Could you check a few things on this model? Use its own coordinates, in mm. Give positions to 0.01 mm unless a question says otherwise; leave off trailing zeros. Use a Markdown table: item, result. Add a question column.
```python
from build123d import *

# Parameters (mm, degrees)
SKETCH_1_W          = 350
SKETCH_1_H          = 310
SKETCH_1_R          = 1.95
SKETCH_1_R_2        = 9
EXTRUDE_1_DEPTH     = 1
SKETCH_2_R          = 2.1
SKETCH_2_R_2        = 1.6
SKETCH_2_R_3        = 11
SKETCH_2_R_4        = 1.5
SKETCH_2_W          = 10
SKETCH_2_H          = 10
CUT_EXTRUDE_1_DEPTH = 10
SKETCH_3_RX         = 29.354112179
SKETCH_3_RY         = 16.489205711
CUT_EXTRUDE_2_DEPTH = 8


with BuildPart() as part:
    # 草图1 → 凸台-拉伸1 (new body)
    with BuildSketch(Plane.XY):
        with Locations((175, 155)):
            Rectangle(SKETCH_1_W, SKETCH_1_H)
        with Locations((10, 300)):
            Circle(SKETCH_1_R, mode=Mode.SUBTRACT)
        with Locations((10, 230)):
            Circle(SKETCH_1_R, mode=Mode.SUBTRACT)
        with Locations((10, 40)):
            Circle(SKETCH_1_R, mode=Mode.SUBTRACT)
        with Locations((10, 10)):
            Circle(SKETCH_1_R, mode=Mode.SUBTRACT)
        with Locations((340, 300)):
            Circle(SKETCH_1_R, mode=Mode.SUBTRACT)
        with Locations((340, 230)):
            Circle(SKETCH_1_R, mode=Mode.SUBTRACT)
        with Locations((340, 40)):
            Circle(SKETCH_1_R, mode=Mode.SUBTRACT)
        with Locations((340, 10)):
            Circle(SKETCH_1_R, mode=Mode.SUBTRACT)
        with Locations((130, 10)):
            Circle(SKETCH_1_R, mode=Mode.SUBTRACT)
        with Locations((220, 10)):
            Circle(SKETCH_1_R, mode=Mode.SUBTRACT)
        with Locations((10, 160)):
            Circle(SKETCH_1_R, mode=Mode.SUBTRACT)
        with Locations((340, 160)):
            Circle(SKETCH_1_R, mode=Mode.SUBTRACT)
        with Locations((130, 162)):
            Circle(SKETCH_1_R, mode=Mode.SUBTRACT)
        with Locations((220, 162)):
            Circle(SKETCH_1_R, mode=Mode.SUBTRACT)
        with Locations((175, 280)):
            Circle(SKETCH_1_R_2, mode=Mode.SUBTRACT)
        with Locations((130, 182)):
            Circle(SKETCH_1_R, mode=Mode.SUBTRACT)
        with Locations((220, 182)):
            Circle(SKETCH_1_R, mode=Mode.SUBTRACT)
        with Locations((80, 240)):
            Circle(SKETCH_1_R, mode=Mode.SUBTRACT)
        with Locations((270, 240)):
            Circle(SKETCH_1_R, mode=Mode.SUBTRACT)
        with Locations((155, 280)):
            Circle(SKETCH_1_R, mode=Mode.SUBTRACT)
        with Locations((195, 280)):
            Circle(SKETCH_1_R, mode=Mode.SUBTRACT)
    extrude(amount=EXTRUDE_1_DEPTH)

    # 草图2 → 切除-拉伸1 (cut)
    with BuildSketch(Plane(origin=(0, 0, 0), x_dir=(-1, 0, 0), z_dir=(0, 0, -1))):
        with Locations((-130, 135)):
            Circle(SKETCH_2_R)
        with Locations((-220, 45)):
            Circle(SKETCH_2_R)
        with Locations((-220, 135)):
            Circle(SKETCH_2_R)
        with Locations((-130, 45)):
            Circle(SKETCH_2_R)
        with Locations((-153.079689783, 50)):
            Circle(SKETCH_2_R_2)
        with Locations((-175, 28.079689783)):
            Circle(SKETCH_2_R_2)
        with Locations((-196.920310217, 50)):
            Circle(SKETCH_2_R_2)
        with Locations((-175, 50)):
            Circle(SKETCH_2_R_3)
        with Locations((-150, 137)):
            Circle(SKETCH_2_R_4)
        with Locations((-135, 90)):
            Circle(SKETCH_2_R_3)
        with Locations((-200, 137)):
            Circle(SKETCH_2_R_4)
        with Locations((-113.079689783, 90)):
            Circle(SKETCH_2_R_2)
        with Locations((-135, 68.079689783)):
            Circle(SKETCH_2_R_2)
        with Locations((-135, 111.920310217)):
            Circle(SKETCH_2_R_2)
        with Locations((-175, 110)):
            Rectangle(SKETCH_2_W, SKETCH_2_H)
    extrude(amount=-CUT_EXTRUDE_1_DEPTH, mode=Mode.SUBTRACT)

    # 草图3 → 切除-拉伸2 (cut)
    with BuildSketch(Plane.XY.offset(1)):
        with Locations((175, 244.534964975)):
            Ellipse(SKETCH_3_RX, SKETCH_3_RY)
    extrude(amount=-CUT_EXTRUDE_2_DEPTH, mode=Mode.SUBTRACT)


solid = part.part
```
1) For pin 1 (4.5 mm diameter, centred on x = 220, y = 10, fed in from +Z), with a flat end and sliding along its axis, tell me the tip position at first contact or that it passes through.
2) Please list where these lines run through material, in increasing order: line 1 (Y direction, x = 340, z = 0.5); line 2 (X direction, y = 50.5, z = 0.95); line 3 (X direction, y = 160, z = 0.1). Write a range as from..to.
3) Suppose I cut it at A-A on z = 0.5. Count the separate pieces of the cut face and the enclosed holes in it, and give its area (3 significant figures).
4) We'd pull the mould along X, two halves only. Please class faces 1 (the face through (185.99, 50.48, 0.49)), 2 (the face through (173, 157, 0)): pulls with the +X half, pulls with the -X half, needs draft (parallel to the pull), parting line crosses it, or undercut.
Values found:
| question | item | result |
|---|---|---|
| 1 | pin 1 | stops at z = 1 |
| 2 | line 1 | y = 0..8.05, 11.95..38.05, 41.95..158.05, 161.95..228.05, 231.95..298.05, 301.95..310 |
| 2 | line 2 | x = 0..151.56, 154.6..164.01, 185.99..195.4, 198.44..350 |
| 2 | line 3 | x = 0..8.05, 11.95..338.05, 341.95..350 |
| 3 | separate pieces | 1 |
| 3 | enclosed holes | 37 |
| 3 | area | 106,000 mm^2 |
| 4 | face 1 | undercut |
| 4 | face 2 | needs draft |
